from build123d import *

# Parameters (mm, degrees)
FILLET1_R           = 3
BOSS_EXTRUDE2_DEPTH = 0.5
CIRPATTERN3_COUNT   = 3


with BuildPart() as part:
    # Sketch1 → Revolve2 (revolve)
    with BuildSketch(Plane(origin=(0, 0, 0), x_dir=(0, 0, -1), z_dir=(1, 0, 0))):
        Polygon((6.835567607, 0), (6.835567607, 4.933028396), (56.835567607, 4.933028396), (56.835567607, 6.266802226), (-11.993527317, 6.266802226), (-11.993527317, 10.876596073), (-30.238642963, 3.628152456), (-33.164432393, 0), align=None)
    revolve(axis=Axis((0, 0, 44.67851679), (0, 0, -1)))

    # Fillet1
    fillet1_edges = [part.edges().sort_by_distance(p)[0] for p in [
        (0, -6.266802226, 11.993527317),
    ]]
    fillet(fillet1_edges, radius=FILLET1_R)

    # Sketch2 → Boss-Extrude2 (add, symmetric)
    with BuildSketch(Plane(origin=(0, 0, 0), x_dir=(1, 0, 0), z_dir=(0, 1, 0))):
        Polygon((5.575190906, 1.997056238), (18.315636179, 57.181987564), (5.575190906, 57.181987564), align=None)
    boss_extrude2 = extrude(amount=BOSS_EXTRUDE2_DEPTH, both=True)

    # CirPattern3: Boss-Extrude2 ×3 about axis
    cirpattern3_axis = Axis((0, 0, 0), (0, 0, 1))
    for i in range(1, CIRPATTERN3_COUNT):
        add(boss_extrude2.rotate(cirpattern3_axis, i * 360 / CIRPATTERN3_COUNT))


solid = part.part
Design review of the part built by this model. Coordinates are the model's own, in mm. A direction names the side the tool comes from. Give positions to 0.01 mm unless a question says otherwise; leave off trailing zeros. Order: outer loops, then holes, each group sorted by start corner. A loop starts at its lowest first (then second) coordinate and runs counter-clockwise, first axis right, second up. Notation, with made-up numbers: (77.5, -9) - (120.5, -9) arc R21 ccw to (120.5, -1) - close; hole circle Ø10 at (-31.75, 46.25). An arc over 180 degrees is marked (long way). Write item = value, one per line. Start each with the question number.
Q1. To check wall thickness, follow L1, parallel to Y at x = -4, z = -42; L2, parallel to X at y = 0, z = -17; L3, parallel to Y at x = -2.5, z = -27.5. State the ranges of each line that lie inside material, in increasing order. Write a range as from..to.
Q2. Tool access review of faces 5 (the face through (12.2, 0, -30.7)), 6 (the face through (-6.09, -10.57, -30.68)), 7 (the face through (-4.816, -1.069, -32.186)): name each direction out of +Z, -Z, +X, -X, +Y, -Y from which nothing blocks a thin tool from reaching the whole face with its end or side.
Q3. We need section D-D on x = 12.25. State the section outline as (y, z) points.
Q4. We need section A-A on z = -23.5. State the section outline as (x, y) points.
Q5. Mouldability with a two-part tool opening along Y and no side actions: class faces 1 (the face through (-5.65, 8.79, -43.03)), 2 (the face through (0.17, 0.55, 32.7)), 3 (the face through (-5, 2, -56.836)), 4 (the face through (-4.787, -9.292, -43.027)) as released by +Y, released by -Y, zero draft, split by the parting line, or undercut.
Q6. We need section C-C on z = -50. State the section outline as (x, y) points.
Q7. Clearance check with flat-ended pins moving along their axes: pin 1 Ø1.5 at (x, y) = (10, 6) entering from +Z; pin 2 Ø2 at (x, y) = (-3.5, -0.5) entering from +Z; pin 3 Ø10 at (x, z) = (9, -38.5) entering from -Y; pin 4 Ø4 at (y, z) = (-2.5, 0) entering from +X. State where each tip first meets the part, or that it passes through.
Q8. We need section B-B on y = 13. State the section outline as (x, z) points.
Working result:
q1.L1 = -7.93..-5.93, -4.82..-2.89, 2.89..4.82, 5.93..7.93
q1.L2 = -6.27..-4.93, 4.93..9.04
q1.L3 = -5.75..-4.25, 4.25..5.75
q2.face_5 = +X, +Y, -Y
q2.face_6 = -X, -Y
q2.face_7 = -Z
q3.outline = (-0.5, -57.18) - (0.5, -57.18) - (0.5, -30.91) - (-0.5, -30.91) - close
q4.outline = (-5.7, -8.88) - (-4.84, -9.38) - (-2.69, -5.66) arc R6.27 ccw to (6.25, -0.5) - (10.54, -0.5) - (10.54, 0.5) - (6.25, 0.5) arc R6.27 ccw to (-2.69, 5.66) - (-4.84, 9.38) - (-5.7, 8.88) - (-3.56, 5.16) arc R6.27 ccw to (-3.56, -5.16) - close; hole circle Ø9.87 at (0, 0)
q5.face_1 = undercut
q5.face_2 = split by the parting line
q5.face_3 = undercut
q5.face_4 = released by -Y
q6.outline = (-8.76, -14.18) - (-7.9, -14.68) - (-2.69, -5.66) arc R6.27 ccw to (6.25, -0.5) - (16.66, -0.5) - (16.66, 0.5) - (6.25, 0.5) arc R6.27 ccw to (-2.69, 5.66) - (-7.9, 14.68) - (-8.76, 14.18) - (-3.56, 5.16) arc R6.27 ccw to (-3.56, -5.16) - close; hole circle Ø9.87 at (0, 0)
q7.pin_1 = through
q7.pin_2 = 31.12
q7.pin_3 = -4.82
q7.pin_4 = 6.25
q8.outline = (-8.08, -57.18) - (-6.93, -57.18) - (-6.93, -41.62) - (-8.08, -44.12) - close
